Could you check a few things on this model? Use its own coordinates, in mm. A direction names the side the tool comes from. Round coordinates to 2 decimals unless told otherwise and drop trailing zeros. Write each loop counter-clockwise with the first axis right and the second up, starting at its lowest first coordinate (ties: lowest second). Pieces come first, ordered by that corner, then holes. Notation, with made-up numbers: (-27, 73) -> (3, 73) arc R26 cw to (3, 110) -> close; hole circle Ø9 at (46.5, -29). An arc over 180 degrees is marked (long way). Answer in a Markdown table with one row per item.
from build123d import *

# Parameters (mm, degrees)
F1_DEPTH  = 16
F3_DEPTH  = 25
F4_SIZE   = 1
F11_ANGLE = 180
F14_DEPTH = 2
F16_DEPTH = 2


with BuildPart() as f1:
    # F0 (on Right) → F1 (new body)
    with BuildSketch(Plane.YZ):
        with BuildLine():
            Line((0, 7), (0, 0))
            Line((0, 0), (150, 0))
            Line((150, 0), (150, 7))
            ThreePointArc((150, 7), (148.5355339059, 10.5355339059), (145, 12))
            Line((145, 12), (128.050036002, 10.517070303))
            Line((128.050036002, 10.517070303), (127.1432693018, 20.8814611121))
            Line((127.1432693018, 20.8814611121), (113.1965435286, 19.6612807136))
            Line((113.1965435286, 19.6612807136), (113.8937894705, 11.6917231289))
            Line((113.8937894705, 11.6917231289), (5.5800139851, 2.2154956702))
            Line((5.5800139851, 2.2154956702), (4.9427024368, 9.5))
            Line((4.9427024368, 9.5), (20, 9.5))
            Line((20, 9.5), (20, 12))
            Line((20, 12), (5, 12))
            ThreePointArc((5, 12), (1.4644660941, 10.5355339059), (0, 7))
        make_face()
    extrude(amount=F1_DEPTH)

    # F2 (on face) → F3 (cut)
    with BuildSketch(Plane(origin=(0, 114.0437613881, 9.9775362673), x_dir=(1, 0, 0), z_dir=(0, -0.9961946981, -0.0871557427))):
        with BuildLine():
            Line((6, 9.7207347769), (6, 6.8026639789))
            ThreePointArc((6, 6.8026639789), (8, 2.6707347769), (10, 6.8026639789))
            Line((10, 6.8026639789), (10, 9.7207347769))
            Line((10, 9.7207347769), (11.5, 9.7207347769))
            ThreePointArc((11.5, 9.7207347769), (12.2071067812, 9.4278415581), (12.5, 8.7207347769))
            Line((12.5, 8.7207347769), (12.5, 4.7207347769))
            ThreePointArc((12.5, 4.7207347769), (13.3786796564, 2.5994144334), (15.5, 1.7207347769))
            Line((15.5, 1.7207347769), (18.5, 1.7207347769))
            Line((18.5, 1.7207347769), (18.5, 10.7207347769))
            Line((18.5, 10.7207347769), (-2.5, 10.7207347769))
            Line((-2.5, 10.7207347769), (-2.5, 1.7207347769))
            Line((-2.5, 1.7207347769), (0.5, 1.7207347769))
            ThreePointArc((0.5, 1.7207347769), (2.6213203436, 2.5994144334), (3.5, 4.7207347769))
            Line((3.5, 4.7207347769), (3.5, 8.7207347769))
            ThreePointArc((3.5, 8.7207347769), (3.7928932188, 9.4278415581), (4.5, 9.7207347769))
            Line((4.5, 9.7207347769), (6, 9.7207347769))
        make_face()
    extrude(amount=-F3_DEPTH, mode=Mode.SUBTRACT)

    # F4
    f4_edges = [f1.edges().sort_by_distance(p)[0] for p in [
        (6, 120.169906, 20.271371),
        (10, 120.169906, 20.271371),
    ]]
    chamfer(f4_edges, length=F4_SIZE)


with BuildPart() as f5_1:
    # F5: copy of F1
    add(f1.part.moved(Location((32, 0, 0))))


with BuildPart() as f6_1:
    # F6: copy of F5_1
    add(f5_1.part.moved(Location((32, 0, 0))))


with BuildPart() as f7_1:
    # F7: copy of F1
    add(f1.part.moved(Location((0, 160, 0))))


with BuildPart() as f8_1:
    # F8: copy of F5_1
    add(f5_1.part.moved(Location((0, 160, 0))))


with BuildPart() as f9_1:
    # F9: copy of F6_1
    add(f6_1.part.moved(Location((0, 160, 0))))


with BuildPart() as f8_1_1:
    # F11: moved
    add(f8_1.part.rotate(Axis((0, 0, 25), (0, 0, 1)), F11_ANGLE))


with BuildPart() as f9_1_1:
    # F11: moved
    add(f9_1.part.rotate(Axis((0, 0, 25), (0, 0, 1)), F11_ANGLE))


with BuildPart() as f7_1_1:
    # F11: moved
    add(f7_1.part.rotate(Axis((0, 0, 25), (0, 0, 1)), F11_ANGLE))


with BuildPart() as f7_1_2:
    # F12: moved
    add(f7_1_1.part.moved(Location((96, 310, 0))))

    # F13 (on face) → F14 (join)
    with BuildSketch(Plane.YZ.offset(96)):
        with BuildLine():
            Line((0, 7), (0, 0))
            Line((0, 0), (150, 0))
            Line((150, 0), (150, 7))
            ThreePointArc((150, 7), (148.5355339059, 10.5355339059), (145, 12))
            Line((145, 12), (5, 12))
            ThreePointArc((5, 12), (1.4644660941, 10.5355339059), (0, 7))
        make_face()
    extrude(amount=F14_DEPTH)


with BuildPart() as f8_1_2:
    # F12: moved
    add(f8_1_1.part.moved(Location((96, 310, 0))))


with BuildPart() as f9_1_2:
    # F12: moved
    add(f9_1_1.part.moved(Location((96, 310, 0))))


with BuildPart() as f1_1:
    add(f1.part)

    add(f5_1.part)  # F16 merges F5_1

    add(f6_1.part)  # F16 merges F6_1

    add(f7_1_2.part)  # F16 merges F7_1

    add(f8_1_2.part)  # F16 merges F8_1

    add(f9_1_2.part)  # F16 merges F9_1
    # F15 (on face) → F16 (join)
    with BuildSketch(Plane(origin=(0, 0, 0), x_dir=(0, -1, 0), z_dir=(-1, 0, 0))):
        with BuildLine():
            Line((-150, 0), (0, 0))
            Line((0, 0), (0, 7))
            ThreePointArc((0, 7), (-1.4644660941, 10.5355339059), (-5, 12))
            Line((-5, 12), (-145, 12))
            ThreePointArc((-145, 12), (-148.5355339059, 10.5355339059), (-150, 7))
            Line((-150, 7), (-150, 0))
        make_face()
    extrude(amount=F16_DEPTH)


solid = f1_1.part
1) Imagine slicing it at D-D, the plane y = 42. Please give me the cut outline in (x, z), plus the area to 3 significant figures.
Findings:
| item | result |
|---|---|
| outline | (-2, 0) -> (98, 0) -> (98, 12) -> (96, 12) -> (96, 11.18) -> (80, 11.18) -> (80, 5.4) -> (64, 5.4) -> (64, 11.18) -> (48, 11.18) -> (48, 5.4) -> (32, 5.4) -> (32, 11.18) -> (16, 11.18) -> (16, 5.4) -> (0, 5.4) -> (0, 12) -> (-2, 12) -> close |
| area | 844 mm^2 |
2) Imagine slicing it at B-B, the plane y = 13. Please give me the cut outline in (x, z), plus the area to 3 significant figures.
Findings:
| item | result |
|---|---|
| outline | (-2, 0) -> (98, 0) -> (98, 12) -> (96, 12) -> (96, 11.3) -> (80, 11.3) -> (80, 12) -> (64, 12) -> (64, 11.3) -> (48, 11.3) -> (48, 12) -> (32, 12) -> (32, 11.3) -> (16, 11.3) -> (16, 12) -> (-2, 12) -> close; hole (0, 2.86) -> (16, 2.86) -> (16, 9.5) -> (0, 9.5) -> close; hole (32, 2.86) -> (48, 2.86) -> (48, 9.5) -> (32, 9.5) -> close; hole (64, 2.86) -> (80, 2.86) -> (80, 9.5) -> (64, 9.5) -> close |
| area | 848 mm^2 |
3) Thinking about a two-plate mould opening in X: for faces 1 (the face through (24, 137, 12)), 2 (the face through (88, 138, 9.5)), which applies, +X half, -X half, draft (parallel to the pull), parting line (faces both ways), or undercut?
Findings:
| item | result |
|---|---|
| face 1 | draft |
| face 2 | undercut |
4) Imagine slicing it at C-C, the plane x = 88.5. Please give me the cut outline in (y, z).
Findings:
| item | result |
|---|---|
| outline | (0, 0) -> (150, 0) -> (150, 7) arc R5 ccw to (145, 12) -> (130, 12) -> (130, 9.5) -> (145.06, 9.5) -> (144.42, 2.22) -> (36.11, 11.69) -> (36.19, 12.69) -> (22.25, 13.91) -> (21.95, 10.52) -> (5, 12) arc R5 ccw to (0, 7) -> close |
5) For pin 1 (3.5 mm diameter, centred on y = 123, z = 18, fed in from -X); pin 2 (8 mm diameter, centred on y = 15.5, z = 18.5, fed in from -X); pin 3 (2 mm diameter, centred on x = 17.5, y = 56.5, fed in from +Z) (3 decimals); pin 4 (2.5 mm diameter, centred on y = 121, z = 17, fed in from +X), each with a flat end and sliding along its axis, tell me the tip position at first contact or that it passes through.
Findings:
| item | result |
|---|---|
| pin 1 | stops at x = 3.5 |
| pin 2 | passes through |
| pin 3 | stops at z = 9.995 |
| pin 4 | stops at x = 76.5 |
6) Imagine slicing it at A-A, the plane z = 5.5. Please give me the cut outline in (x, y), plus the area to 3 significant figures.
Findings:
| item | result |
|---|---|
| outline | (-2, 0) -> (98, 0) -> (98, 150) -> (-2, 150) -> close; hole (0, 5.29) -> (16, 5.29) -> (16, 43.12) -> (0, 43.12) -> close; hole (16, 106.88) -> (32, 106.88) -> (32, 144.71) -> (16, 144.71) -> close; hole (32, 5.29) -> (48, 5.29) -> (48, 43.12) -> (32, 43.12) -> close; hole (48, 106.88) -> (64, 106.88) -> (64, 144.71) -> (48, 144.71) -> close; hole (64, 5.29) -> (80, 5.29) -> (80, 43.12) -> (64, 43.12) -> close; hole (80, 106.88) -> (96, 106.88) -> (96, 144.71) -> (80, 144.71) -> close |
| area | 11,400 mm^2 |
7) Please list where these lines run through material, in increasing order: line 1 (X direction, y = 48, z = 6.5); line 2 (X direction, y = 55, z = 11); line 3 (Z direction, x = 4.5, y = 37.5).
Findings:
| item | result |
|---|---|
| line 1 | x = -2 to 0, 16 to 32, 48 to 64, 80 to 98 |
| line 2 | x = -2 to 0, 96 to 98 |
| line 3 | z = 0 to 5.01 |
8) For faces 3 (the face through (96, 101, 8)), 4 (the face through (7.89, 136.64, 11.27)), 5 (the face through (56, 137, 12)), 6 (the face through (22, 30, 18)), which set-ups out of +Z, -Z, +X, -X, +Y, -Y let a thin tool reach every point of the face, with its end or its side?
Findings:
| item | result |
|---|---|
| face 3 | none |
| face 4 | +Z |
| face 5 | +Z, +X, -X, +Y |
| face 6 | +Z, +Y, -Y |
